```python
from build123d import *

# Parameters (mm, degrees)
F0_W     = 2000
F0_H     = 500
F1_DEPTH = 500
F2_W     = 1900
F2_H     = 450
F3_DEPTH = 500.001
F4_W     = 400
F4_H     = 400
F5_DEPTH = 2000.001
F6_SCALE = 0.5


with BuildPart() as f1:
    # F0 (on Front) → F1 (new body)
    with BuildSketch(Plane.XZ):
        with Locations((1000, 250)):
            Rectangle(F0_W, F0_H)
    extrude(amount=F1_DEPTH)

    # F2 (on face) → F3 (cut, through all)
    with BuildSketch(Plane.XZ.offset(500)):
        with Locations((1000, 225)):
            Rectangle(F2_W, F2_H)
    extrude(amount=-F3_DEPTH, mode=Mode.SUBTRACT)

    # F4 (on face) → F5 (cut, through all)
    with BuildSketch(Plane(origin=(0, 0, 0), x_dir=(0, -1, 0), z_dir=(-1, 0, 0))):
        with Locations((250, 250)):
            Rectangle(F4_W, F4_H)
    extrude(amount=-F5_DEPTH, mode=Mode.SUBTRACT)


with BuildPart() as f1_1:
    # F6: moved
    add(f1.part.scale(F6_SCALE))


solid = f1_1.part
```
Could you check a few things on this model? Use its own coordinates, in mm. A direction names the side the tool comes from. Round coordinates to 2 decimals unless told otherwise and drop trailing zeros. Loops run counter-clockwise (first coordinate to the right, second up) from the corner with the lowest first, then second, coordinate; pieces in that order, holes last. Notation, with made-up numbers: (27, -19) - (50, -19) arc R15 cw to (50, -3) - close; hole circle Ø4 at (43.5, -22). An arc over 180 degrees is marked (long way). Answer as CSV lines item,"result".
1. For pin 1 Ø1.5 at (x, y) = (845.5, -100) entering from -Z, with a flat end and sliding along its axis, tell me the tip position at first contact or that it passes through.
Filled in:
pin 1,"stops at z = 225"
2. We'd pull the mould along X, two halves only. Please class faces 1 (the face through (12, -124, 25)), 2 (the face through (0, -123, 234)), 3 (the face through (1000, -123, 234)), 4 (the face through (975, -126, 20)): +X half, -X half, draft (parallel to the pull), parting line (faces both ways), or undercut.
Filled in:
face 1,"draft"
face 2,"-X half"
face 3,"+X half"
face 4,"undercut"
3. Please list where these lines run through material, in increasing order: line 1 along X through (y, z) = (-238, 141); line 2 along Z through (x, y) = (59.5, -46). Write a range as [from, to].
Filled in:
line 1,"x = [0, 25], [975, 1000]"
line 2,"z = [225, 250]"
4. On a 3-axis mill with a long thin cutter (end or side, diameter ignored), from which of +Z, -Z, +X, -X, +Y, -Y can I reach the whole of each face in a straight line? I mean faces 5 (the face through (12, -225, 124)), 6 (the face through (25, -126, 20)), 7 (the face through (12, -123, 0)). Say none if no direction works.
Filled in:
face 5,"+X, -X"
face 6,"-Z, +Y, -Y"
face 7,"-Z, +X, -X, +Y, -Y"
5. I want a section at C-C on x = 764. List the corners of the cut face in (y, z) for me.
Filled in:
outline,"(-250, 225) - (0, 225) - (0, 250) - (-250, 250) - close"
6. I want a section at A-A on y = -194. List the corners of the cut face in (x, z) for me, then the cut area to 4 significant figures.
Filled in:
outline,"(0, 0) - (25, 0) - (25, 25) - (0, 25) - close; (0, 225) - (1000, 225) - (1000, 250) - (0, 250) - close; (975, 0) - (1000, 0) - (1000, 25) - (975, 25) - close"
area,"26,250 mm^2"
7. I want a section at B-B on z = 71. List the corners of the cut face in (x, y) for me, then the cut area to 3 significant figures.
Filled in:
outline,"(0, -250) - (25, -250) - (25, -225) - (0, -225) - close; (0, -25) - (25, -25) - (25, 0) - (0, 0) - close; (975, -250) - (1000, -250) - (1000, -225) - (975, -225) - close; (975, -25) - (1000, -25) - (1000, 0) - (975, 0) - close"
area,"2,500 mm^2"
